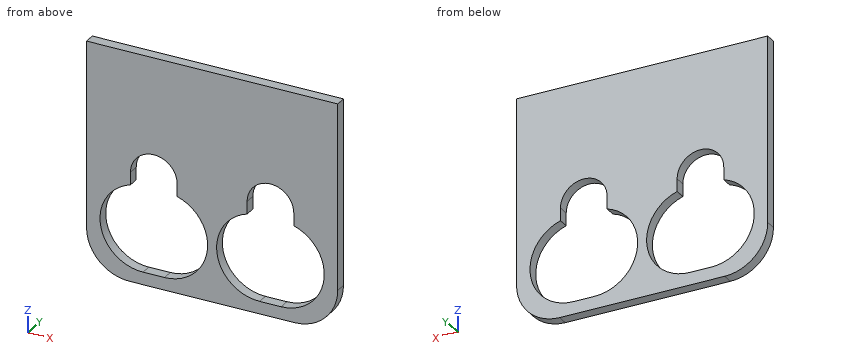
from build123d import *

# Parameters (mm, degrees)
SKETCH1_W               = 70
SKETCH1_H               = 67
BOSS_EXTRUDE1_DEPTH     = 3
SKETCH5_W               = 70
SKETCH5_H               = 3
CUT_EXTRUDE4_DEPTH      = 1
CUT_EXTRUDE4_DEPTH_BACK = 4
FILLET1_R               = 12
CUT_EXTRUDE1_START      = -4
SKETCH2_R               = 6.5
CUT_EXTRUDE1_DEPTH      = 5
CUT_EXTRUDE2_START      = -4
CUT_EXTRUDE2_DEPTH      = 5
CUT_EXTRUDE3_START      = -4
SKETCH4_W               = 13
SKETCH4_H               = 8.828059947
CUT_EXTRUDE3_DEPTH      = 5


with BuildPart() as part:
    # Sketch1 → Boss-Extrude1 (new body)
    with BuildSketch(Plane(origin=(0, 0, 0), x_dir=(1, 0, 0), z_dir=(0, 1, 0))):
        Rectangle(SKETCH1_W, SKETCH1_H)
    extrude(amount=BOSS_EXTRUDE1_DEPTH)

    # Sketch5 → Cut-Extrude4 (cut, two sides)
    with BuildSketch(Plane(origin=(0, 3, 0), x_dir=(1, 0, 0), z_dir=(0, 1, 0))) as cut_extrude4_sk:
        with Locations((0, 32)):
            Rectangle(SKETCH5_W, SKETCH5_H)
    extrude(amount=CUT_EXTRUDE4_DEPTH, mode=Mode.SUBTRACT)
    extrude(cut_extrude4_sk.sketch, amount=-CUT_EXTRUDE4_DEPTH_BACK, mode=Mode.SUBTRACT)

    # Fillet1
    fillet1_edges = [part.edges().sort_by_distance(p)[0] for p in [
        (-35, 1.5, -30.5),
        (35, 1.5, -30.5),
    ]]
    fillet(fillet1_edges, radius=FILLET1_R)

    # Sketch2 → Cut-Extrude1 (cut)
    with BuildSketch(Plane(origin=(0, 3, 0), x_dir=(1, 0, 0), z_dir=(0, 1, 0)).offset(CUT_EXTRUDE1_START)):
        with Locations((-16.25, 0)):
            Circle(SKETCH2_R)
    cut_extrude1 = extrude(amount=CUT_EXTRUDE1_DEPTH, mode=Mode.SUBTRACT)

    # Sketch3 → Cut-Extrude2 (cut)
    with BuildSketch(Plane(origin=(0, 3, 0), x_dir=(1, 0, 0), z_dir=(0, 1, 0)).offset(CUT_EXTRUDE2_START)):
        with BuildLine():
            Line((-19.25, 27), (-13.25, 27))
            ThreePointArc((-13.25, 27), (-1.25, 15), (-13.25, 3))
            Line((-13.25, 3), (-19.25, 3))
            ThreePointArc((-19.25, 3), (-31.25, 15), (-19.25, 27))
        make_face()
    cut_extrude2 = extrude(amount=CUT_EXTRUDE2_DEPTH, mode=Mode.SUBTRACT)

    # Sketch4 → Cut-Extrude3 (cut)
    with BuildSketch(Plane(origin=(0, 3, 0), x_dir=(1, 0, 0), z_dir=(0, 1, 0)).offset(CUT_EXTRUDE3_START)):
        with Locations((-16.25, 4.414029973)):
            Rectangle(SKETCH4_W, SKETCH4_H)
    cut_extrude3 = extrude(amount=CUT_EXTRUDE3_DEPTH, mode=Mode.SUBTRACT)

    # Mirror1: Cut-Extrude1, Cut-Extrude2, Cut-Extrude3 across plane
    add(cut_extrude1.mirror(Plane(origin=(0, 0, 0), x_dir=(0, 0, 1), z_dir=(1, 0, 0))), mode=Mode.SUBTRACT)
    add(cut_extrude2.mirror(Plane(origin=(0, 0, 0), x_dir=(0, 0, 1), z_dir=(1, 0, 0))), mode=Mode.SUBTRACT)
    add(cut_extrude3.mirror(Plane(origin=(0, 0, 0), x_dir=(0, 0, 1), z_dir=(1, 0, 0))), mode=Mode.SUBTRACT)


solid = part.part
The model under review builds one solid part; all positions refer to its coordinate system, in mm. Round coordinates to 2 decimals unless told otherwise and drop trailing zeros. Loops run counter-clockwise (first coordinate to the right, second up) from the corner with the lowest first, then second, coordinate; pieces in that order, holes last. Notation, with made-up numbers: M 26,-23.5 L 39,-23.5 A20 cw 39,5.5 Z; hole C 14,-25.5 d7. An arc over 180 degrees is marked long. Answer as a JSON object with one key per item and string values.
Item 1: We need section D-D, the plane x = 3.5. State the section outline as (y, z) points, and give its area (3 significant figures).
Check sheet entries:
{"outline": "M 0,-30.5 L 3,-30.5 L 3,-22 L 0,-22 Z; M 0,-8 L 3,-8 L 3,33.5 L 0,33.5 Z", "area": "150 mm2"}
Item 2: We need section B-B, the plane y = 2.5. State the section outline as (x, z) points.
Check sheet entries:
{"outline": "M -35,-18.5 A12 ccw -23,-30.5 L 23,-30.5 A12 ccw 35,-18.5 L 35,33.5 L -35,33.5 Z; hole M -22.75,-3.52 A12 ccw -19.25,-27 L -13.25,-27 A12 ccw -9.75,-3.52 L -9.75,0 A6.5 ccw -22.75,0 Z; hole M 9.75,-3.52 A12 ccw 13.25,-27 L 19.25,-27 A12 ccw 22.75,-3.52 L 22.75,0 A6.5 ccw 9.75,0 Z"}
Item 3: We need section A-A, the plane x = -16.25. State the section outline as (y, z) points.
Check sheet entries:
{"outline": "M 0,-30.5 L 3,-30.5 L 3,-27 L 0,-27 Z; M 0,6.5 L 3,6.5 L 3,33.5 L 0,33.5 Z"}
Item 4: For line 1 along X through (y, z) = (0.65, -7.5); line 2 along X through (y, z) = (2.35, 5); line 3 along Z through (x, y) = (7.5, 0.45), list the stretches that pass through material, from the lowest coordinate up.
Check sheet entries:
{"line 1": "-35 to -28.62, -3.88 to 3.88, 28.62 to 35", "line 2": "-35 to -20.4, -12.1 to 12.1, 20.4 to 35", "line 3": "-30.5 to -25.53, -4.47 to 33.5"}
Item 5: We need section C-C, the plane z = -10. State the section outline as (x, y) points, and give its area (3 significant figures).
Check sheet entries:
{"outline": "M -35,0 L -30.16,0 L -30.16,3 L -35,3 Z; M -2.34,0 L 2.34,0 L 2.34,3 L -2.34,3 Z; M 30.16,0 L 35,0 L 35,3 L 30.16,3 Z", "area": "43.1 mm2"}
